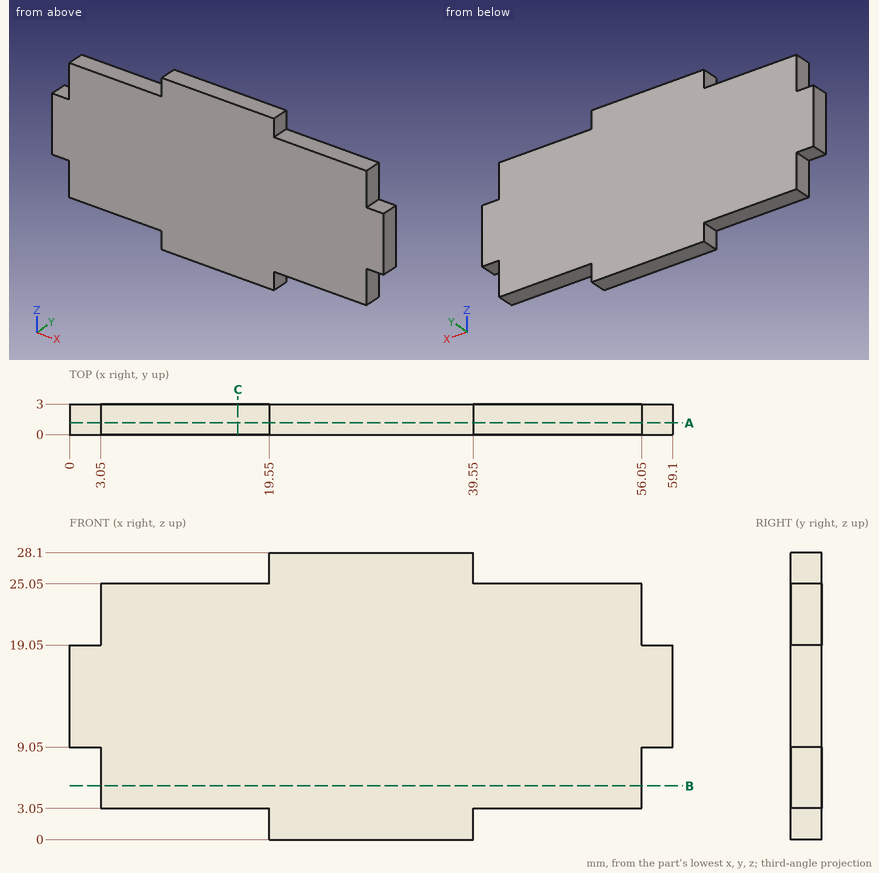
Study the drawing (mm; zero at the part's minimum x, y, z) and answer. Give positions to 0.01 mm unless a question says otherwise; leave off trailing zeros. Order: outer loops, then holes, each group sorted by start corner. A loop starts at its lowest first (then second) coordinate and runs counter-clockwise, first axis right, second up. Notation, with made-up numbers: (74, -38.75) -> (92, -38.75) arc R32 cw to (92, 0.25) -> close; hole circle Ø9 at (-19.5, 46). An arc over 180 degrees is marked (long way). Write item = value, one per line.
1. Straight lines are drawn through the part: line 1 along Z through (x, y) = (43, 2.95); line 2 along X through (y, z) = (1.1, 5.5); line 3 along X through (y, z) = (1.1, 1.75). For each, find the intervals that lie inside material, in ascending order.
Numbers:
line_1 = 3.05 to 25.05
line_2 = 3.05 to 56.05
line_3 = 19.55 to 39.55
2. A cutting plane is placed at A-A, the plane y = 1.15. Write down the section's boundary in (x, z).
Numbers:
outline = (0, 9.05) -> (3.05, 9.05) -> (3.05, 3.05) -> (19.55, 3.05) -> (19.55, 0) -> (39.55, 0) -> (39.55, 3.05) -> (56.05, 3.05) -> (56.05, 9.05) -> (59.1, 9.05) -> (59.1, 19.05) -> (56.05, 19.05) -> (56.05, 25.05) -> (39.55, 25.05) -> (39.55, 28.1) -> (19.55, 28.1) -> (19.55, 25.05) -> (3.05, 25.05) -> (3.05, 19.05) -> (0, 19.05) -> close
3. A cutting plane is placed at C-C, the plane x = 16.5. Write down the section's boundary in (y, z), and give its area (3 significant figures).
Numbers:
outline = (0, 3.05) -> (3, 3.05) -> (3, 25.05) -> (0, 25.05) -> close
area = 66.0 mm²
4. Given pin 1 (0.9 mm diameter, centred on y = 2, z = 1.5, fed in from +X); pin 2 (0.9 mm diameter, centred on x = 10.5, y = 1, fed in from +Z); pin 3 (0.9 mm diameter, centred on x = 57, y = 1, fed in from +Z), each flat-ended and moving along its own axis, determine where each tip first touches the part or whether it passes through.
Numbers:
pin_1 = 39.55
pin_2 = 25.05
pin_3 = 19.05
5. A cutting plane is placed at B-B, the plane z = 5.25. Write down the section's boundary in (x, y).
Numbers:
outline = (3.05, 0) -> (56.05, 0) -> (56.05, 3) -> (3.05, 3) -> close
